```python
from build123d import *

# Parameters (mm, degrees)
F1_DEPTH = 1828.8
F3_SIZE  = 101.6
F4_SIZE  = 101.6


with BuildPart() as f1:
    # F0 (on Right) → F1 (new body)
    with BuildSketch(Plane.YZ):
        Polygon((-1327.777296, 758.974876), (-1700.789874, -307.825124), (-24.389874, -307.825124), (298.899346, 15.464096), (298.899346, 396.464096), (-63.611433, 758.974876), align=None)
    extrude(amount=F1_DEPTH)

    # F3
    f3_edges = [f1.edges().sort_by_distance(p)[0] for p in [
        (1828.8, -695.694365, 758.974876),
    ]]
    chamfer(f3_edges, length=F3_SIZE)

    # F4
    f4_edges = [f1.edges().sort_by_distance(p)[0] for p in [
        (0, -695.694365, 758.974876),
    ]]
    chamfer(f4_edges, length=F4_SIZE)


solid = f1.part
```
Check sheet for the modelled part. Datum: model origin and axes. Units: mm. Give positions to 0.01 mm unless a question says otherwise; leave off trailing zeros. Write each loop counter-clockwise with the first axis right and the second up, starting at its lowest first coordinate (ties: lowest second). Pieces come first, ordered by that corner, then holes.
Item 1: Cross-section at A-A (x = 563). Enter the section's corners in (y, z).
Item 2: Scan lines: L1, parallel to Y at x = 1716, z = -41; L2, parallel to Y at x = 561.5, z = 697; L3, parallel to Z at x = 748.5, y = 32. Record each from-to range of solid material in increasing order.
Item 3: Gauge pin test, flat ends, axial feed: pin 1 (1.5 mm diameter, centred on x = 1571.5, y = 39.5, fed in from -Z); pin 2 (10 mm diameter, centred on x = 542, y = 98, fed in from +Z); pin 3 (4 mm diameter, centred on x = 471.5, z = 504, fed in from +Y). Record the tip position at first contact, or that the pin passes through.
Item 4: Cross-section at B-B (z = 439.5). Enter the section's corners in (x, y), and give its area (3 significant figures).
Item 5: Cross-section at C-C (z = -103). Enter the section's corners in (x, y), and give its area (3 significant figures).
Report:
1. outline: (-1700.79, -307.83) - (-24.39, -307.83) - (298.9, 15.46) - (298.9, 396.46) - (-63.61, 758.97) - (-1327.78, 758.97) - close
2. L1: y = -1607.49 to 242.44
2. L2: y = -1349.45 to -1.64
2. L3: z = -251.44 to 663.36
3. pin 1: stops at z = -244.69
3. pin 2: stops at z = 602.36
3. pin 3: stops at y = 193.36
4. outline: (0, -1439.48) - (1828.8, -1439.48) - (1828.8, 255.86) - (0, 255.86) - close
4. area: 3,100,000 mm2
5. outline: (0, -1629.17) - (1828.8, -1629.17) - (1828.8, 180.44) - (0, 180.44) - close
5. area: 3,310,000 mm2
